Here's the drawing with two shaded views (mm, measured from the low corner). I have some questions. A direction names the side the tool comes from. Give positions to 0.01 mm unless a question says otherwise; leave off trailing zeros. Order: outer loops, then holes, each group sorted by start corner. A loop starts at its lowest first (then second) coordinate and runs counter-clockwise, first axis right, second up. Notation, with made-up numbers: M -1,-31.75 L 13,-31.75 A34 cw 13,0.25 Z; hole C 46.25,63.25 d6. An arc over 180 degrees is marked long. Use a Markdown table: item, result. Add a question column.
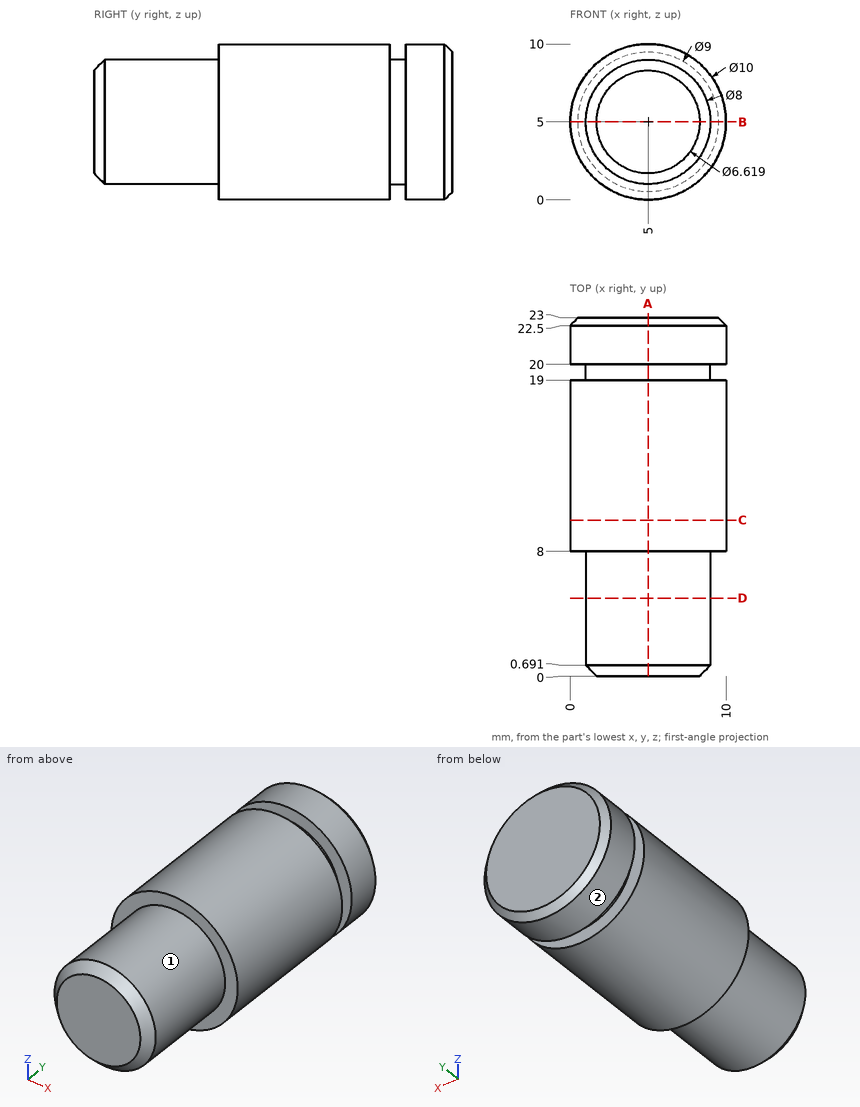
1. If we section it at C-C, the plane y = 10: List the corners of the cut face in (x, z) for me.
2. If we section it at A-A, the plane x = 5: List the corners of the cut face in (y, z) for me.
3. On a 3-axis mill with a long thin cutter (end or side, diameter ignored), from which of +Z, -Z, +X, -X, +Y, -Y can I reach the whole of each face in a straight line? I mean the marked faces 1 and 2. Say none if no direction works.
4. I need wall thicknesses on L1, parallel to Y at x = 4.75, z = 9.25; L2, parallel to X at y = 8.5, z = 8.75 (1 decimal); L3, parallel to Z at x = 8, y = 13.5. Which ranges of each line are inside material? Lowest first, please. Write a range as [from, to].
5. Will these pins go through, and if not, where does the flat tip stop? pin 1 (1 mm diameter, centred on y = 7, z = 5, fed in from +X); pin 2 (4 mm diameter, centred on x = 3.5, y = 2.5, fed in from -Z); pin 3 (4 mm diameter, centred on y = 9, z = 2.5, fed in from +X) (1 decimal).
6. If we section it at D-D, the plane y = 5: List the corners of the cut face in (x, z) for me.
7. If we section it at B-B, the plane z = 5: List the corners of the cut face in (x, y) for me, then the cut area to 3 significant figures.
Geometry results:
| question | item | result |
|---|---|---|
| 1 | outline | C 5,5 d10 |
| 2 | outline | M 0,1.69 L 0.69,1 L 8,1 L 8,0 L 19,0 L 19,1 L 20,1 L 20,0 L 22.5,0 L 23,0.5 L 23,9.5 L 22.5,10 L 20,10 L 20,9 L 19,9 L 19,10 L 8,10 L 8,9 L 0.69,9 L 0,8.31 Z |
| 3 | face 1 | -Y |
| 3 | face 2 | +Y, -Y |
| 4 | L1 | y = [8, 19], [20, 23] |
| 4 | L2 | x = [1.7, 8.3] |
| 4 | L3 | z = [1, 9] |
| 5 | pin 1 | stops at x = 9 |
| 5 | pin 2 | stops at z = 1 |
| 5 | pin 3 | stops at x = 10 |
| 6 | outline | C 5,5 d8 |
| 7 | outline | M 0,8 L 1,8 L 1,0.69 L 1.69,0 L 8.31,0 L 9,0.69 L 9,8 L 10,8 L 10,19 L 9,19 L 9,20 L 10,20 L 10,22.5 L 9.5,23 L 0.5,23 L 0,22.5 L 0,20 L 1,20 L 1,19 L 0,19 Z |
| 7 | area | 211 mm^2 |
